Here's how the part is built. I have some questions about the finished solid (model axes, mm). A direction names the side the tool comes from. Give positions to 0.01 mm unless a question says otherwise; leave off trailing zeros. Loops run counter-clockwise (first coordinate to the right, second up) from the corner with the lowest first, then second, coordinate; pieces in that order, holes last. Notation, with made-up numbers: (76, -34.5) - (119, -34.5) arc R16 ccw to (119, -24.5) - close; hole circle Ø11 at (76, 8). An arc over 180 degrees is marked (long way). Return JSON: item names as keys, results as strings. Group by question number.
(1) If we section it at D-D (x = 10): Please give me the cut outline in (y, z).
(2) If we section it at A-A (x = -66): Please give me the cut outline in (y, z).
(3) On a 3-axis mill with a long thin cutter (end or side, diameter ignored), from which of +Z, -Z, +X, -X, +Y, -Y can I reach the whole of each face in a straight line? I mean faces 1 (the flat face through (-22, 56, 10)), 2 (the cylindrical face through (19.516, 84.375, 19.86)), 3 (the flat face through (-55, 5, 10)). Say none if no direction works.
(4) If we mould it in two halves opening along Y, with no side actions, what happens to faces 4 (the flat face through (22, 56, 10)), 5 (the flat face through (-50, 0, 30)), 6 (the cylindrical face through (67.932, 5.07, 28.959))? For each: released by +Y, released by -Y, zero draft, split by the parting line, or undercut.
(5) I need wall thicknesses on probe 1 along X at (y, z) = (5, 30); probe 2 along Y at (x, z) = (69.5, 25). Which ranges of each line are inside material? Lowest first, please. Write a range as [from, to].
(6) If we section it at C-C (z = 43.5): Please give me the cut outline in (x, y), then the cut area to 3 significant figures.
(7) If we section it at B-B (y = 19.5): Please give me the cut outline in (x, z), then the cut area to 3 significant figures.
(8) For P1, Ø5, axis at y = 34, z = 39, coming from the -X side; P2, Ø9.5, axis at x = -60, z = 30, coming from the +Y side; P3, Ø1, axis at y = 28, z = 31.5, coming from the -X side; P4, Ø4, axis at y = 67, z = 18.5, coming from the -X side, each with a flat end and sliding along its axis, tell me the tip position at first contact or that it passes through.
```python
from build123d import *

# Parameters (mm, degrees)
BOSS_EXTRUDE1_DEPTH  = 60
BOSS_EXTRUDE2_DEPTH  = 30
BOSS_EXTRUDE3_DEPTH  = 10
BOSS_EXTRUDE4_DEPTH  = 10
FILLET1_R            = 10
FILLET1_OF_MIRROR2_R = 10
SKETCH13_R           = 8
CUT_EXTRUDE1_DEPTH   = 135.53624053
RIB1_START           = -5
RIB1_DEPTH           = 10


with BuildPart() as part:
    # Sketch2 → Boss-Extrude1 (new body)
    with BuildSketch(Plane.XY):
        with BuildLine():
            ThreePointArc((-30, 0), (-21.213203436, 21.213203436), (0, 30))
            Line((0, 30), (0, 40))
            ThreePointArc((0, 40), (-28.284271247, 28.284271247), (-40, 0))
            Line((-40, 0), (-30, 0))
        make_face()
        with BuildLine():
            Line((0, 40), (0, 30))
            ThreePointArc((0, 30), (21.213203436, 21.213203436), (30, 0))
            Line((30, 0), (40, 0))
            ThreePointArc((40, 0), (28.284271247, 28.284271247), (0, 40))
        make_face()
    extrude(amount=BOSS_EXTRUDE1_DEPTH)



with BuildPart() as body_2:
    # Sketch2<3> → Boss-Extrude2 (new body)
    with BuildSketch(Plane.XY):
        with BuildLine():
            Line((-25, 100), (-15, 100))
            ThreePointArc((-15, 100), (0, 85), (15, 100))
            Line((15, 100), (25, 100))
            ThreePointArc((25, 100), (0, 75), (-25, 100))
        make_face()
    extrude(amount=BOSS_EXTRUDE2_DEPTH)


with BuildPart() as part_1:
    add(part.part)

    add(body_2.part)  # Boss-Extrude3 merges body 2
    # Sketch8 → Boss-Extrude3 (add)
    with BuildSketch(Plane(origin=(0, 0, 0), x_dir=(-1, 0, 0), z_dir=(0, 0, -1))):
        with BuildLine():
            Line((-25, 100), (-39.529411765, 6.117647059))
            ThreePointArc((-39.529411765, 6.117647059), (0, 40), (39.529411765, 6.117647059))
            Line((39.529411765, 6.117647059), (25, 100))
            ThreePointArc((25, 100), (0, 75), (-25, 100))
        make_face()
    extrude(amount=-BOSS_EXTRUDE3_DEPTH)

    # Sketch10 → Boss-Extrude4 (add)
    with BuildSketch(Plane.XZ):
        with BuildLine():
            Line((35, 50), (60, 50))
            ThreePointArc((60, 50), (80, 30), (60, 10))
            Line((60, 10), (35, 10))
            Line((35, 10), (35, 50))
        make_face()
    boss_extrude4 = extrude(amount=-BOSS_EXTRUDE4_DEPTH)

    # Fillet1
    fillet1_edges = [part_1.edges().sort_by_distance(p)[0] for p in [
        (39.228991597, 8.058823529, 10),
        (39.88217942, 3.067859955, 10),
        (39.681187851, 5.040171699, 50),
    ]]
    fillet(fillet1_edges, radius=FILLET1_R - 0.0001)  # a hair under: the kernel refuses the full size

    # Mirror2: Boss-Extrude4 across plane
    add(boss_extrude4.mirror(Plane(origin=(0, 0, 0), x_dir=(0, 0, 1), z_dir=(1, 0, 0))))

    # Fillet1 of Mirror2
    fillet1_of_mirror2_edges = [part_1.edges().sort_by_distance(p)[0] for p in [
        (-39.228991597, 8.058823529, 10),
        (-39.88217942, 3.067859955, 10),
        (-39.681187851, 5.040171699, 50),
    ]]
    fillet(fillet1_of_mirror2_edges, radius=FILLET1_OF_MIRROR2_R - 0.0001)  # a hair under: the kernel refuses the full size

    # Sketch13 → Cut-Extrude1 (cut, through all)
    with BuildSketch(Plane(origin=(0, 10, 0), x_dir=(1, 0, 0), z_dir=(0, 1, 0))):
        with Locations(Location((60, -30, 0), (0, 0, 270))):
            Circle(SKETCH13_R)
        with Locations(Location((-60, -30, 0), (0, 0, 270))):
            Circle(SKETCH13_R)
    extrude(amount=-CUT_EXTRUDE1_DEPTH, mode=Mode.SUBTRACT)

    # Rib1: read off the stored shape, not the designer's step
    # Rib1 outline → Rib1 (add)
    with BuildSketch(Plane(origin=(0, 0, 0), x_dir=(0, 0, -1), z_dir=(1, 0, 0)).offset(RIB1_START)):
        Polygon((-60, 40), (-60, 39.686269666), (-10, 39.686269666), (-10, 75.505102572), (-30, 75.505102572), (-30, 75), align=None)
    extrude(amount=RIB1_DEPTH)


solid = part_1.part
```
Values:
{
 "1": {"outline": "(28.28, 0) - (88.82, 0) - (88.82, 30) - (77.09, 30) - (77.09, 10) - (38.73, 10) - (38.73, 60) - (28.28, 60) - close"},
 "2": {"outline": "(0, 10.92) - (10, 10.92) - (10, 24.71) - (0, 24.71) - close; (0, 35.29) - (10, 35.29) - (10, 49.08) - (0, 49.08) - close"},
 "3": {"face 1": "+Z, -X", "face 2": "+Z, +X", "face 3": "-Z, -X, +Y, -Y"},
 "4": {"face 4": "undercut", "face 5": "released by -Y", "face 6": "zero draft"},
 "5": {"probe 1": "[-80, -68], [-52, -29.58], [29.58, 52], [68, 80]", "probe 2": "[0, 10]"},
 "6": {"outline": "(-74.76, 0) - (-30, 0) arc R30 cw to (30, 0) - (74.76, 0) - (74.76, 10) - (38.73, 10) arc R40 ccw to (5, 39.69) - (5, 59.25) - (-5, 59.25) - (-5, 39.69) arc R40 ccw to (-38.73, 10) - (-74.76, 10) - close", "area": "2,000 mm2"},
 "7": {"outline": "(-37.46, 0) - (-22.8, 0) - (-22.8, 60) - (-34.92, 60) - (-34.92, 10) - (-37.46, 10) - close; (22.8, 0) - (37.46, 0) - (37.46, 10) - (34.92, 10) - (34.92, 60) - (22.8, 60) - close", "area": "1,510 mm2"},
 "8": {"P1": "x = -24.65", "P2": "through", "P3": "x = -29.05", "P4": "x = -5"}
}
